from build123d import *

# Parameters (mm, degrees)
SKETCH1_W                                = 82.55
SKETCH1_H                                = 50.8
BOSS_EXTRUDE1_DEPTH                      = 45.466
SKETCH2_R                                = 14
CUT_EXTRUDE1_DEPTH                       = 51.8
F_5_32_0_15625_DIAMETER_HOLE1_AT_2_COUNT = 2
F_5_32_0_15625_DIAMETER_HOLE1_AT_2_PITCH = 42.8625
F_5_32_0_15625_DIAMETER_HOLE1_AT_3_COUNT = 2
F_5_32_0_15625_DIAMETER_HOLE1_AT_3_PITCH = 49.823226574
F_5_32_0_15625_DIAMETER_HOLE1_AT_4_COUNT = 2
F_5_32_0_15625_DIAMETER_HOLE1_AT_4_PITCH = 25.4
TAP_DRILL_FOR_3_8_24_TAP2_D              = 8.4328
TAP_DRILL_FOR_3_8_24_TAP2_DEPTH          = 31.75
TAP_DRILL_FOR_3_8_24_TAP2_TIP            = 2.533468714


with BuildPart() as part:
    # Sketch1 → Boss-Extrude1 (new body)
    with BuildSketch(Plane.XY):
        with Locations((41.275, 25.4)):
            Rectangle(SKETCH1_W, SKETCH1_H)
    extrude(amount=BOSS_EXTRUDE1_DEPTH)

    # Sketch2 → Cut-Extrude1 (cut, through all)
    with BuildSketch(Plane(origin=(0, 50.8, 0), x_dir=(1, 0, 0), z_dir=(0, 1, 0))):
        with Locations((27.813, -23.241)):
            Circle(SKETCH2_R)
    extrude(amount=-CUT_EXTRUDE1_DEPTH, mode=Mode.SUBTRACT)

    # Sketch6 → 5/32 (0.15625) Diameter Hole1 (revolve, cut)
    with BuildSketch(Plane(origin=(6.35, 38.1, 45.466), x_dir=(0, -1, 0), z_dir=(1, 0, 0))):
        Polygon((0, 0), (0, 13.892332791), (1.984375, 12.7), (1.984375, 0), align=None)
    f_5_32_0_15625_diameter_hole1 = revolve(axis=Axis((6.35, 38.1, 51.816), (0, 0, -1)), mode=Mode.SUBTRACT)

    # 5/32 (0.15625) Diameter Hole1 at 2: 5/32 (0.15625) Diameter Hole1 ×2
    with Locations(*[(i * F_5_32_0_15625_DIAMETER_HOLE1_AT_2_PITCH, 0, 0) for i in range(1, F_5_32_0_15625_DIAMETER_HOLE1_AT_2_COUNT)]):
        add(f_5_32_0_15625_diameter_hole1, mode=Mode.SUBTRACT)

    # 5/32 (0.15625) Diameter Hole1 at 3: 5/32 (0.15625) Diameter Hole1 ×2
    with Locations(*[Vector(0.860291534, -0.50980239, 0) * (i * F_5_32_0_15625_DIAMETER_HOLE1_AT_3_PITCH) for i in range(1, F_5_32_0_15625_DIAMETER_HOLE1_AT_3_COUNT)]):
        add(f_5_32_0_15625_diameter_hole1, mode=Mode.SUBTRACT)

    # 5/32 (0.15625) Diameter Hole1 at 4: 5/32 (0.15625) Diameter Hole1 ×2
    with Locations(*[(0, -i * F_5_32_0_15625_DIAMETER_HOLE1_AT_4_PITCH, 0) for i in range(1, F_5_32_0_15625_DIAMETER_HOLE1_AT_4_COUNT)]):
        add(f_5_32_0_15625_diameter_hole1, mode=Mode.SUBTRACT)

    # Mirror1: 5/32 (0.15625) Diameter Hole1 across plane
    add(f_5_32_0_15625_diameter_hole1.mirror(Plane.XY.offset(22.733)), mode=Mode.SUBTRACT)

    # Mirror1 copy 1 sketch → Mirror1 copy 1 (revolve, cut)
    with BuildSketch(Plane(origin=(49.2125, 38.1, 0), x_dir=(0, -1, 0), z_dir=(1, 0, 0))):
        Polygon((0, 0), (0, -13.892332791), (1.984375, -12.7), (1.984375, 0), align=None)
    revolve(axis=Axis((49.2125, 38.1, -6.35), (0, 0, -1)), mode=Mode.SUBTRACT)

    # Mirror1 copy 2 sketch → Mirror1 copy 2 (revolve, cut)
    with BuildSketch(Plane(origin=(49.2125, 12.7, 0), x_dir=(0, -1, 0), z_dir=(1, 0, 0))):
        Polygon((0, 0), (0, -13.892332791), (1.984375, -12.7), (1.984375, 0), align=None)
    revolve(axis=Axis((49.2125, 12.7, -6.35), (0, 0, -1)), mode=Mode.SUBTRACT)

    # Mirror1 copy 3 sketch → Mirror1 copy 3 (revolve, cut)
    with BuildSketch(Plane(origin=(6.35, 12.7, 0), x_dir=(0, -1, 0), z_dir=(1, 0, 0))):
        Polygon((0, 0), (0, -13.892332791), (1.984375, -12.7), (1.984375, 0), align=None)
    revolve(axis=Axis((6.35, 12.7, -6.35), (0, 0, -1)), mode=Mode.SUBTRACT)

    # Tap Drill for 3/8-24 Tap2
    with Locations(Plane(origin=(0, 0, 0), x_dir=(-1, 0, 0), z_dir=(0, -1, 0))):
        with Locations((-74.295, -23.241)):
            Hole(TAP_DRILL_FOR_3_8_24_TAP2_D / 2, depth=TAP_DRILL_FOR_3_8_24_TAP2_DEPTH)
            with Locations((0, 0, -(TAP_DRILL_FOR_3_8_24_TAP2_DEPTH + TAP_DRILL_FOR_3_8_24_TAP2_TIP / 2))):  # 118° drill point
                Cone(0, TAP_DRILL_FOR_3_8_24_TAP2_D / 2, TAP_DRILL_FOR_3_8_24_TAP2_TIP, mode=Mode.SUBTRACT)


solid = part.part
The model under review builds one solid part; all positions refer to its coordinate system, in mm. A direction names the side the tool comes from. Round coordinates to 2 decimals unless told otherwise and drop trailing zeros. Loops run counter-clockwise (first coordinate to the right, second up) from the corner with the lowest first, then second, coordinate; pieces in that order, holes last. Notation, with made-up numbers: (-37, 41) -> (9, 41) arc R20 cw to (9, 61) -> close; hole circle Ø5 at (88, -20). An arc over 180 degrees is marked (long way). Return JSON: item names as keys, results as strings.
(1) Add section A-A on z = 34. Write out the cut boundary in (x, y), plus the area to 3 significant figures.
Solved:
{"outline": "(0, 0) -> (18.86, 0) -> (18.86, 50.8) -> (0, 50.8) -> close; (36.77, 0) -> (82.55, 0) -> (82.55, 50.8) -> (36.77, 50.8) -> close; hole circle Ø3.97 at (6.35, 12.7); hole circle Ø3.97 at (6.35, 38.1); hole circle Ø3.97 at (49.21, 12.7); hole circle Ø3.97 at (49.21, 38.1)", "area": "3,230 mm2"}
(2) Add section C-C on x = 28.5. Write out the cut boundary in (y, z), plus the area to 3 significant figures.
Solved:
{"outline": "(0, 0) -> (50.8, 0) -> (50.8, 9.26) -> (0, 9.26) -> close; (0, 37.22) -> (50.8, 37.22) -> (50.8, 45.47) -> (0, 45.47) -> close", "area": "889 mm2"}
(3) For line 1 (X direction, y = 12.7, z = 3.25); line 2 (Y direction, x = 6.35, z = 8.75); line 3 (X direction, y = 28.5, z = 21.5), list the stretches that pass through material, from the lowest coordinate up.
Solved:
{"line 1": "0 to 4.37, 8.33 to 47.23, 51.2 to 82.55", "line 2": "0 to 10.72, 14.68 to 36.12, 40.08 to 50.8", "line 3": "0 to 13.92, 41.7 to 70.45, 78.14 to 82.55"}
(4) The part is to be moulded in two halves that separate along Z. For faces 4 (the flat face through (41, 26, 0)), 5 (the cylindrical face through (70.083, 16.097, 23.056)), 6 (the cylindrical face through (5.009, 14.163, 39.205)), say which applies: released by +Z, released by -Z, zero draft, split by the parting line, or undercut.
Solved:
{"face 4": "released by -Z", "face 5": "undercut", "face 6": "zero draft"}
(5) For pin 1 (3.5 mm diameter, centred on x = 6.35, y = 12.7, fed in from +Z); pin 2 (3 mm diameter, centred on x = 49.21, y = 12.7, fed in from -Z), all flat-tipped, find the tip position at first contact; note any pin that passes through.
Solved:
{"pin 1": "z = 32.63", "pin 2": "z = 12.99"}
(6) Add section B-B on x = 19. Write out the cut boundary in (y, z), plus the area to 3 significant figures.
Solved:
{"outline": "(0, 0) -> (50.8, 0) -> (50.8, 12.36) -> (0, 12.36) -> close; (0, 34.12) -> (50.8, 34.12) -> (50.8, 45.47) -> (0, 45.47) -> close", "area": "1,200 mm2"}
(7) For faces 1 (the cylindrical face through (40.745, 25.756, 28.603)), 2 (the cylindrical face through (50.42, 14.275, 39.205)), 3 (the cylindrical face through (6.263, 14.682, 6.261)), list the 3-axis set-ups (+Z, -Z, +X, -X, +Y, -Y) from which the entire face can be reached by the end or side of a thin tool; tool diameter is ignored.
Solved:
{"face 1": "+Y, -Y", "face 2": "+Z", "face 3": "-Z"}
